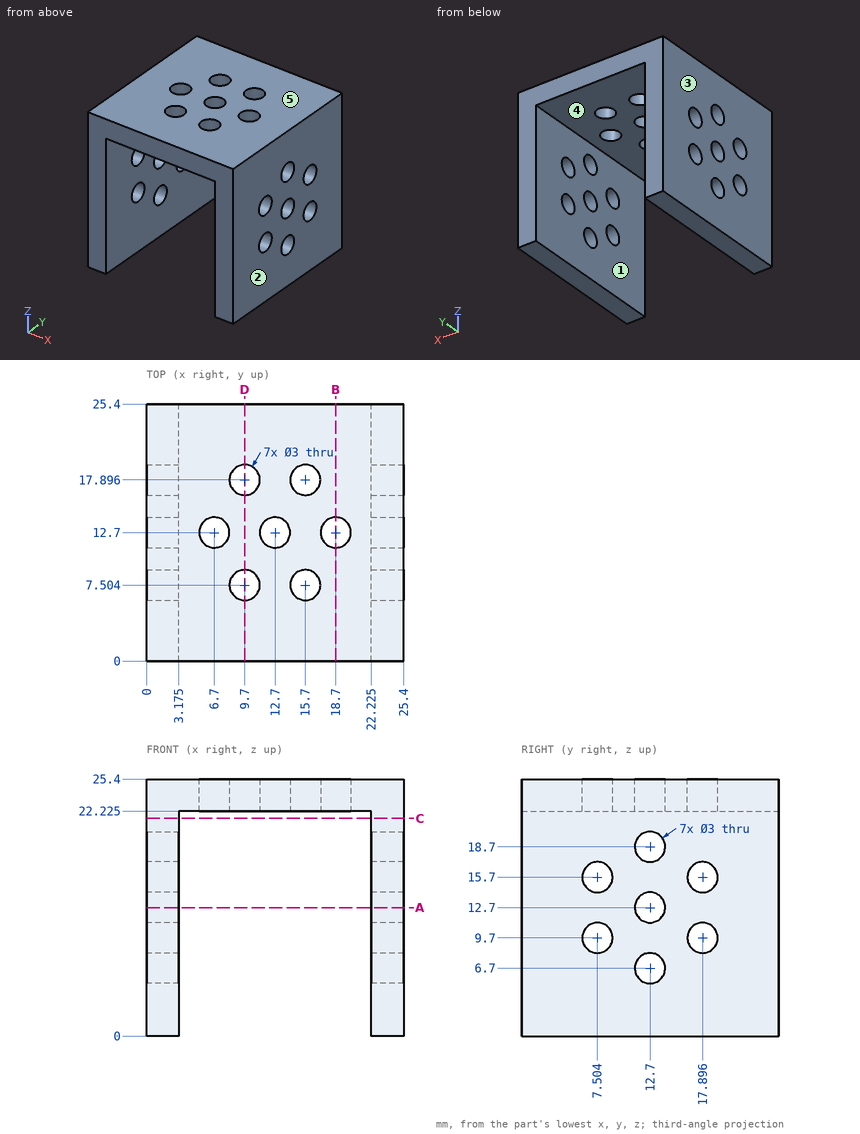
Study the drawing (mm; zero at the part's minimum x, y, z) and answer. A direction names the side the tool comes from. Coordinates: 2 decimals unless noted, no trailing zeros. Loops run counter-clockwise (first coordinate to the right, second up) from the corner with the lowest first, then second, coordinate; pieces in that order, holes last. Notation, with made-up numbers: (28, -26.5) -> (69, -26.5) arc R25 cw to (69, -7.5) -> close; hole circle Ø3 at (-13.5, 30). An arc over 180 degrees is marked (long way). Write each question's results on one line, items separated by ' | '. Start each with the question number.
1) Consider line 1 along Y through (x, z) = (9.7, 23.5); line 2 along X through (y, z) = (20, 18) (3 decimals); line 3 along Y through (x, z) = (23.3, 12.7). Determine where each line is inside the solid, lowest interval first.
2) The mould has two halves that part along X. Classify the marked faces 1, 2 and 3: pulls with the +X half, pulls with the -X half, needs draft (parallel to the pull), parting line crosses it, or undercut.
3) Find section A-A on z = 12.7. Determine the outline of the cut face in (x, y) (3 decimals).
4) For the marked faces 4 and 5, determine the directions among +Z, -Z, +X, -X, +Y, -Y from which every point of the face is accessible in a straight line to the end or side of a thin tool.
5) Find section B-B on x = 18.7. Determine the outline of the cut face in (y, z) (3 decimals), then the cut area to 3 significant figures.
6) Find section D-D on x = 9.7. Determine the outline of the cut face in (y, z) (3 decimals).
7) Find section C-C on z = 21.5. Determine the outline of the cut face in (x, y) (3 decimals), then the cut area to 3 significant figures.
8) Flat-ended cylindrical pins translate along their axes: P1, Ø4, axis at x = 9.7, y = 17.9, coming from the +Z side; P2, Ø3.5, axis at x = 15.7, y = 17.9, coming from the -Z side (3 decimals). Find the tip coordinate at first contact, or state that the pin passes through.
Response values:
1) line 1: y = 0 to 6, 9 to 16.4, 19.4 to 25.4 | line 2: x = 0 to 3.175, 22.225 to 25.4 | line 3: y = 0 to 11.2, 14.2 to 25.4
2) face 1: undercut | face 2: pulls with the +X half | face 3: pulls with the -X half
3) outline: (0, 0) -> (3.175, 0) -> (3.175, 11.2) -> (0, 11.2) -> close; (0, 14.2) -> (3.175, 14.2) -> (3.175, 25.4) -> (0, 25.4) -> close; (22.225, 0) -> (25.4, 0) -> (25.4, 11.2) -> (22.225, 11.2) -> close; (22.225, 14.2) -> (25.4, 14.2) -> (25.4, 25.4) -> (22.225, 25.4) -> close
4) face 4: -Z, +Y, -Y | face 5: +Z, +X, -X, +Y, -Y
5) outline: (0, 22.225) -> (11.2, 22.225) -> (11.2, 25.4) -> (0, 25.4) -> close; (14.2, 22.225) -> (25.4, 22.225) -> (25.4, 25.4) -> (14.2, 25.4) -> close | area: 71.1 mm^2
6) outline: (0, 22.225) -> (6.004, 22.225) -> (6.004, 25.4) -> (0, 25.4) -> close; (9.004, 22.225) -> (16.396, 22.225) -> (16.396, 25.4) -> (9.004, 25.4) -> close; (19.396, 22.225) -> (25.4, 22.225) -> (25.4, 25.4) -> (19.396, 25.4) -> close
7) outline: (0, 0) -> (3.175, 0) -> (3.175, 25.4) -> (0, 25.4) -> close; (22.225, 0) -> (25.4, 0) -> (25.4, 25.4) -> (22.225, 25.4) -> close | area: 161 mm^2
8) P1: stops at z = 25.4 | P2: stops at z = 22.225
